from build123d import *

# Parameters (mm, degrees)
F1_DEPTH = 63.5
F2_DEPTH = 7.9375
F0_W     = 25.341231811
F0_H     = 19.05
F3_DEPTH = 25.4
F5_R     = 6.35
F6_R     = 15.2361087042
F7_DEPTH = 28.575


with BuildPart() as f1:
    # F0 (on Front) → F1 (new body, symmetric)
    with BuildSketch(Plane.XZ):
        Polygon((-41.275, 9.525), (-41.275, -9.525), (41.275, -9.525), (41.275, 9.525), (22.225, 9.525), align=None)
    extrude(amount=F1_DEPTH, both=True)

    # F0 (on Front) → F2 (join, symmetric)
    with BuildSketch(Plane.XZ):
        with BuildLine():
            add(Edge.make_bspline(
                [(-41.275, 9.525), (-41.6624008036, 52.7132268151), (24.7713242394, 61.4626114939), (56.3040405334, 61.9149530076)],
                knots=[0, 0, 0, 0, 110.5062466574, 110.5062466574, 110.5062466574, 110.5062466574], degree=3))
            Line((-41.275, 9.525), (22.225, 9.525))
            Line((22.225, 9.525), (22.225, 27.0002))
            ThreePointArc((22.225, 27.0002), (32.1569933844, 51.3949790585), (56.3040405334, 61.9149530076))
        make_face()
    extrude(amount=F2_DEPTH, both=True)

    # F0 (on Front) → F3 (join, symmetric)
    with BuildSketch(Plane.XZ):
        with BuildLine():
            Line((22.225, 9.525), (41.275, 9.525))
            Line((41.275, 9.525), (41.275, 27.0002))
            ThreePointArc((41.275, 27.0002), (45.9246798487, 38.2255201513), (57.15, 42.8752))
            Line((57.15, 42.8752), (60.325, 42.8752))
            Line((60.325, 42.8752), (60.325, 61.9252))
            Line((60.325, 61.9252), (57.15, 61.9252))
            add(Edge.make_bspline(
                [(56.3040405334, 61.9149530076), (56.5889002651, 61.9190393629), (56.8709117518, 61.9224486028), (57.15, 61.9252)],
                knots=[110.5062466574, 110.5062466574, 110.5062466574, 110.5062466574, 111.5045361635, 111.5045361635, 111.5045361635, 111.5045361635], degree=3))
            ThreePointArc((56.3040405334, 61.9149530076), (32.1569933844, 51.3949790585), (22.225, 27.0002))
            Line((22.225, 27.0002), (22.225, 9.525))
        make_face()
        with Locations((72.9956159055, 52.4002)):
            Rectangle(F0_W, F0_H)
    extrude(amount=F3_DEPTH, both=True)

    # F0 (on Front) → F4 (revolve)
    with BuildSketch(Plane.XZ):
        Polygon((85.666231811, 66.675), (85.666231811, 61.9252), (85.666231811, 42.8752), (85.666231811, 38.1), (111.125, 38.1), (111.125, 66.675), align=None)
    revolve(axis=Axis((85.666231811, 0, 52.3875), (0, 0, -1)))

    # F5
    f5_edges = [f1.edges().sort_by_distance(p)[0] for p in [
        (-41.275, -63.5, 0),
        (41.275, -63.5, 0),
        (41.275, 63.5, 0),
        (-41.275, 63.5, 0),
    ]]
    fillet(f5_edges, radius=F5_R)

    # F6 (on face) → F7 (cut)
    with BuildSketch(Plane(origin=(0, 0, 38.1), x_dir=(1, 0, 0), z_dir=(0, 0, -1))):
        with Locations((85.666231811, 0)):
            Circle(F6_R)
    extrude(amount=-F7_DEPTH, mode=Mode.SUBTRACT)


solid = f1.part
Read the model definition and answer for the solid it produces. Units are mm, in the model's axes. A direction names the side the tool comes from. Round coordinates to 2 decimals unless told otherwise and drop trailing zeros. Write each loop counter-clockwise with the first axis right and the second up, starting at its lowest first coordinate (ties: lowest second). Pieces come first, ordered by that corner, then holes. Notation, with made-up numbers: (36.25, -5) - (89.25, -5) arc R27 cw to (89.25, 15) - close; hole circle Ø4 at (43.5, 43). An arc over 180 degrees is marked (long way). Use a Markdown table: item, result.
(1) The part is cut by section B-B (y = -48). Write down the section's boundary in (x, z) (3 decimals), then the cut area to 3 significant figures.
Reported:
| item | result |
|---|---|
| outline | (-41.275, -9.525) - (41.275, -9.525) - (41.275, 9.525) - (-41.275, 9.525) - close |
| area | 1,570 mm2 |
(2) Each of these flat-tipped pins is pushed along its axis until it touches: pin 1 Ø12 at (y, z) = (-8.5, 42) entering from -X; pin 2 Ø15.5 at (x, z) = (43.5, 30.5) entering from -Y; pin 3 Ø13.5 at (x, y) = (70, 3.5) entering from -Z. Where does it stop, or does it pass through?
Reported:
| item | result |
|---|---|
| pin 1 | x = -30.47 |
| pin 2 | y = -25.4 |
| pin 3 | z = 38.1 |
(3) Straight lines are drawn through the part: line 1 along Z through (x, y) = (73.5, -22) (3 decimals); line 2 along Y through (x, z) = (62.5, 59); line 3 along Z through (x, y) = (1.5, 21.5) (3 decimals). For each, find the intervals that lie inside material, in ascending order. Write a range as [from, to].
Reported:
| item | result |
|---|---|
| line 1 | [38.1, 66.675] |
| line 2 | [-25.4, 25.4] |
| line 3 | [-9.525, 9.525] |
(4) The mould has two halves that part along Y. Classify faces 1 (the cylindrical face through (39.464, 61.59, 0.133)), 2 (the flat face through (1, 35, 9.525)), 3 (the cylindrical face through (99.74, 5.84, 52.19)), 4 (the cylindrical face through (39.464, -61.59, 0.133)): released by +Y, released by -Y, zero draft, split by the parting line, or undercut.
Reported:
| item | result |
|---|---|
| face 1 | released by +Y |
| face 2 | zero draft |
| face 3 | undercut |
| face 4 | released by -Y |
(5) The part is cut by section A-A (x = 62). Write down the section's boundary in (y, z) (3 decimals).
Reported:
| item | result |
|---|---|
| outline | (-25.4, 42.875) - (-9.384, 42.875) - (-9.384, 38.1) - (9.384, 38.1) - (9.384, 42.875) - (25.4, 42.875) - (25.4, 61.925) - (9.384, 61.925) - (9.384, 66.675) - (-9.384, 66.675) - (-9.384, 61.925) - (-25.4, 61.925) - close |
(6) Which of the six approach directions +Z, -Z, +X, -X, +Y, -Y give full straight-line access (tool end or side, diameter ignored) to faces 5 (the cylindrical face through (45.8, -0.4, 38.1)), 6 (the flat face through (22.225, 17, 18)), 7 (the flat face through (41.275, -1, 4))?
Reported:
| item | result |
|---|---|
| face 5 | -Z, +Y, -Y |
| face 6 | +Z, -X, +Y |
| face 7 | -Z, +X, +Y, -Y |
